Model file for the job. Use its own axes, mm. A direction names the side the tool comes from. Give positions to 0.01 mm unless a question says otherwise; leave off trailing zeros. Order: outer loops, then holes, each group sorted by start corner. A loop starts at its lowest first (then second) coordinate and runs counter-clockwise, first axis right, second up. Notation, with made-up numbers: M 34.25,3.5 L 89.25,3.5 A19 cw 89.25,36.5 Z; hole C -21,56.5 d6. An arc over 180 degrees is marked long. Return JSON: item names as keys, results as strings. Group by question number.
1. Two-plate mould, pull along Y, no slides. Class faces 6 (the face through (3.84, 8.57, -0.76)), 7 (the face through (-1.27, 0.97, 1.48)), 8 (the face through (9.014, 1.346, 11.619)), 9 (the face through (0, -4.75, -1)): released by +Y, released by -Y, zero draft, split by the parting line, or undercut.
2. Pin check, flat tips, straight feed: pin 1 (8 mm diameter, centred on x = 1.5, z = 10, fed in from +Y); pin 2 (4 mm diameter, centred on x = 8, z = 6.5, fed in from +Y); pin 3 (1 mm diameter, centred on x = 4.5, y = -3.5, fed in from -Z). Stop position of each tip, or through.
3. Slice it at C-C on z = 11.5. List the corners of the cut face in (x, y), then the cut area to 3 significant figures.
4. Slice it at B-B on y = -10. List the corners of the cut face in (x, z), then the cut area to 3 significant figures.
5. Wall check: probe 1 along X at (y, z) = (7.5, 4.5); probe 2 along Y at (x, z) = (0, 1.75); probe 3 along Z at (x, y) = (0, -11.3). Give the ranges that are in metal, low to high. Write a range as [from, to].
6. Slice it at D-D on z = 15.75. List the corners of the cut face in (x, y).
7. Slice it at A-A on x = 0. List the corners of the cut face in (y, z), then the cut area to 3 significant figures.
8. 3-axis set-ups, long thin cutter, end or side, ignore diameter. For faces 1 (the face through (0, -12.5, 7)), 2 (the face through (-2, 0, 0)), 3 (the face through (0, 4.75, -1)), 4 (the face through (4, -9.5, 12)), 5 (the face through (-8.986, 1.346, 11.619)): which of +Z, -Z, +X, -X, +Y, -Y reach the whole face in a straight line?
from build123d import *

# Parameters (mm, degrees)
SKETCH_W        = 20
SKETCH_H        = 25
PAD_DEPTH       = 3
SKETCH001_W     = 20
SKETCH001_H     = 3
PAD001_DEPTH    = 17
PAD002_DEPTH    = 25
SKETCH003_R     = 1.6
POCKET_DEPTH    = 21.501
SKETCH004_W     = 9.5
SKETCH004_H     = 9.5
POCKET001_DEPTH = 1.5
PAD003_DEPTH    = 20
SKETCH006_W     = 16
SKETCH006_H     = 17
POCKET002_DEPTH = 22
SKETCH007_R     = 3.25
POCKET003_DEPTH = 3.001


with BuildPart() as part:
    # Sketch → Pad (new body)
    with BuildSketch(Plane.XY):
        Rectangle(SKETCH_W, SKETCH_H)
    extrude(amount=PAD_DEPTH)

    # Sketch001 (on Face6 of Pad) → Pad001 (join)
    with BuildSketch(Plane.XY.offset(3)):
        with Locations((0, -11)):
            Rectangle(SKETCH001_W, SKETCH001_H)
    extrude(amount=PAD001_DEPTH)

    # Sketch002 (on Face6 of Pad001) → Pad002 (join)
    with BuildSketch(Plane.XZ.offset(12.5)):
        Polygon((4.75, 0), (-4.75, 0), (-2.95, -1.5), (2.95, -1.5), align=None)
    extrude(amount=-PAD002_DEPTH)

    # Sketch003 (on Face12 of Pad002) → Pocket (cut, through all)
    with BuildSketch(Plane(origin=(0, 0, -1.5), x_dir=(1, 0, 0), z_dir=(0, 0, -1))):
        Circle(SKETCH003_R)
    extrude(amount=-POCKET_DEPTH, mode=Mode.SUBTRACT)

    # Sketch004 (on Face12 of Pocket) → Pocket001 (cut)
    with BuildSketch(Plane(origin=(0, 0, -1.5), x_dir=(1, 0, 0), z_dir=(0, 0, -1))):
        Rectangle(SKETCH004_W, SKETCH004_H)
    extrude(amount=-POCKET001_DEPTH, mode=Mode.SUBTRACT)

    # Sketch005 (on Face3 of Pocket001) → Pad003 (join)
    with BuildSketch(Plane.YZ.offset(10)):
        Polygon((-9.5, 3), (-9.5, 20), (12.5, 3), align=None)
    extrude(amount=-PAD003_DEPTH)

    # Sketch006 (on Face1 of Pad003) → Pocket002 (cut)
    with BuildSketch(Plane(origin=(0, 12.5, 0), x_dir=(-1, 0, 0), z_dir=(0, 1, 0))):
        with Locations((0, 11.5)):
            Rectangle(SKETCH006_W, SKETCH006_H)
    extrude(amount=-POCKET002_DEPTH, mode=Mode.SUBTRACT)

    # Sketch007 (on Face23 of Pocket002) → Pocket003 (cut, through all)
    with BuildSketch(Plane(origin=(0, -9.5, 0), x_dir=(-1, 0, 0), z_dir=(0, 1, 0))):
        with Locations((0, 11.5)):
            Circle(SKETCH007_R)
    extrude(amount=-POCKET003_DEPTH, mode=Mode.SUBTRACT)


solid = part.part
Result:
{
 "1": {"face 6": "zero draft", "face 7": "undercut", "face 8": "released by +Y", "face 9": "undercut"},
 "2": {"pin 1": "stops at y = -9.5", "pin 2": "stops at y = 10.56", "pin 3": "stops at z = 0"},
 "3": {"outline": "M -10,-12.5 L -3.25,-12.5 L -3.25,-9.5 L -8,-9.5 L -8,1.5 L -10,1.5 Z; M 3.25,-12.5 L 10,-12.5 L 10,1.5 L 8,1.5 L 8,-9.5 L 3.25,-9.5 Z", "area": "84.5 mm2"},
 "4": {"outline": "M -10,0 L -4.75,0 L -2.95,-1.5 L 2.95,-1.5 L 4.75,0 L 10,0 L 10,20 L -10,20 Z; hole C 0,11.5 d6.5", "area": "378 mm2"},
 "5": {"probe 1": "x = [-10, -8], [8, 10]", "probe 2": "y = [-12.5, -1.6], [1.6, 12.5]", "probe 3": "z = [-1.5, 8.25], [14.75, 20]"},
 "6": {"outline": "M -10,-12.5 L 10,-12.5 L 10,-4 L 8,-4 L 8,-9.5 L -8,-9.5 L -8,-4 L -10,-4 Z"},
 "7": {"outline": "M -12.5,-1.5 L -4.75,-1.5 L -4.75,0 L -1.6,0 L -1.6,3 L -9.5,3 L -9.5,8.25 L -12.5,8.25 Z; M -12.5,14.75 L -9.5,14.75 L -9.5,20 L -12.5,20 Z; M 1.6,0 L 4.75,0 L 4.75,-1.5 L 12.5,-1.5 L 12.5,3 L 1.6,3 Z", "area": "120 mm2"},
 "8": {"face 1": "+Z, -Z, +X, -X, -Y", "face 2": "-Z", "face 3": "-Z, +X, -X", "face 4": "+Z, +Y", "face 5": "+Z, +X, -X, +Y"}
}
